Input: part model. Units: mm. Frame: model coordinates. A direction names the side the tool comes from. Coordinates: 2 decimals unless noted, no trailing zeros. Write each loop counter-clockwise with the first axis right and the second up, starting at its lowest first coordinate (ties: lowest second). Pieces come first, ordered by that corner, then holes. Notation, with made-up numbers: M 61,64.5 L 95,64.5 A13 ccw 95,87.5 Z; hole C -2,-23.75 d11. An arc over 180 degrees is marked long. Write each question's results on one line, items separated by ' | '. Start each with the question number.
1. Set-up query: faces 4 (the flat face through (64, 110, 54)), 5 (the flat face through (110, 66, 54)), 6 (the cylindrical face through (25, 95, 135)), 7 (the flat face through (10, 20, 54)), 8 (the flat face through (20, 64, 54)). Return all of +Z, -Z, +X, -X, +Y, -Y with unobstructed straight access to the full face (end or side cutting, diameter ignored); none if empty.
2. Pull-direction query (Z, two-part tool) for faces 1 (the flat face through (0, 10, 54)), 2 (the flat face through (64, 66, 140)), 3 (the cylindrical face through (40.024, 63.901, 119.86)); classes: +Z half, -Z half, draft (parallel to the pull), parting line (faces both ways), or undercut.
3. Section query D-D, the plane y = 65. Output: boundary loops of the cut face in (x, z).
4. Section query B-B, the plane x = 33. Output: boundary loops of the cut face in (y, z).
5. Section query C-C, the plane y = 31. Output: boundary loops of the cut face in (x, z).
6. First-contact query: pin 1 (10 mm diameter, centred on y = 42, z = 101.5, fed in from +X); pin 2 (6 mm diameter, centred on x = 120.5, z = 29.5, fed in from +Y); pin 3 (3 mm diameter, centred on x = 79.5, z = 103, fed in from +Y). Flat tips, straight axial feed; report the tip coordinate or a pass-through.
7. Ray query, probe 1 along Z at (x, y) = (90, 26); probe 2 along X at (y, z) = (89.5, 85); probe 3 along Y at (x, z) = (105, 106.5). Return the intervals inside material, ascending.
8. Section query A-A, the plane z = 89.5. Output: boundary loops of the cut face in (x, y), and give its area (3 significant figures).
Autodesk Inventor part; units mm, degrees
ref_plane "YZ Plane" through (0, 0, 0) normal (1, 0, 0) x (0, 1, 0)
ref_plane "XZ Plane" through (0, 0, 0) normal (0, 1, 0) x (-1, 0, 0)
ref_plane "XY Plane" through (0, 0, 0) normal (0, 0, 1) x (1, 0, 0)
sketch "Sketch1" plane through (0, 0, 0) normal (0, 0, 1) x (1, 0, 0)
  line L0 (0, 0) -> (0, 20)
  line L1 (0, 20) -> (20, 20)
  line L2 (20, 20) -> (20, 110)
  line L3 (20, 110) -> (110, 110)
  line L4 (110, 110) -> (110, 20)
  line L5 (110, 20) -> (130, 20)
  line L6 (130, 20) -> (130, 0)
  line L7 (130, 0) -> (0, 0)
  dimension "d0" = 20
  dimension "d1" = 110
  dimension "d2" = 90
  dimension "d3" = 130
extrude "Extrusion1" add sketch "Sketch1" along normal blind 110
sketch "Sketch2" plane through (0, 0, 110) normal (0, 0, 1) x (1, 0, 0)
  line L0 (110, 110) -> (20, 110)
  line L1 (0, 0) -> (130, 0)
  circle A0 centre (65, 65) radius 25
  line L2 (65, 65) -> (65, 0) construction
  line L3 (0, 0) -> (130, 0) construction
  dimension "d6" = 65
  dimension "d7" = 50
extrude "Extrusion2" add sketch "Sketch2" along normal blind 20
sketch "Sketch3" plane through (65, 65, 130) normal (0, 0, 1) x (1, 0, 0)
  circle A0 centre (0, 0) radius 50
  circle A1 centre (0, 0) radius 25
  point P0 (-65, -65)
  dimension "d10" = 100
extrude "Extrusion3" add sketch "Sketch3" along normal blind 10 contours A0 | A1
properties part number "A_Gearbox"
Answer:
1) face 4: -Z, +X, -X, +Y | face 5: -Z, +X, +Y | face 6: +Z | face 7: +Z, -Z, -X, +Y | face 8: -Z, -X, +Y
2) face 1: draft | face 2: +Z half | face 3: undercut
3) outline: M 15,130 L 40,130 L 40,110 L 20,110 L 20,0 L 110,0 L 110,110 L 90,110 L 90,130 L 115,130 L 115,140 L 15,140 Z
4) outline: M 0,0 L 110,0 L 110,110 L 0,110 Z; M 26.58,130 L 103.42,130 L 103.42,140 L 26.58,140 Z
5) outline: M 20,0 L 110,0 L 110,110 L 20,110 Z; M 28.34,130 L 101.66,130 L 101.66,140 L 28.34,140 Z
6) pin 1: x = 110 | pin 2: y = 20 | pin 3: y = 110
7) probe 1: 0 to 110, 130 to 140 | probe 2: 20 to 110 | probe 3: 0 to 110
8) outline: M 0,0 L 130,0 L 130,20 L 110,20 L 110,110 L 20,110 L 20,20 L 0,20 Z | area: 10,700 mm^2
